CAD build for the part. Positions are in the model's coordinates, mm. Face numbers are marked on the shaded views. A direction names the side the tool comes from. Give positions to 0.01 mm unless a question says otherwise; leave off trailing zeros. Loops run counter-clockwise (first coordinate to the right, second up) from the corner with the lowest first, then second, coordinate; pieces in that order, holes last. Notation, with made-up numbers: (51.5, 64.25) - (91.5, 64.25) arc R17 ccw to (91.5, 92.25) - close; hole circle Ø1 at (55.25, 37.25). An arc over 180 degrees is marked (long way). Return JSON: item names as keys, results as strings.
from build123d import *

# Parameters (mm, degrees)
SKETCH1_R           = 6
SKETCH1_R_2         = 2.4
BOSS_EXTRUDE1_DEPTH = 20
SKETCH2_R           = 3.9
CUT_EXTRUDE1_DEPTH  = 7.5
CUT_EXTRUDE2_START  = -10
CUT_EXTRUDE2_DEPTH  = 10
FILLET1_R           = 1


with BuildPart() as part:
    # Sketch1 → Boss-Extrude1 (new body)
    with BuildSketch(Plane.XY):
        Circle(SKETCH1_R)
        Circle(SKETCH1_R_2, mode=Mode.SUBTRACT)
    extrude(amount=BOSS_EXTRUDE1_DEPTH)

    # Sketch2 → Cut-Extrude1 (cut)
    with BuildSketch(Plane.XY.offset(20)):
        Circle(SKETCH2_R)
    extrude(amount=-CUT_EXTRUDE1_DEPTH, mode=Mode.SUBTRACT)

    # Sketch4 → Cut-Extrude2 (cut)
    with BuildSketch(Plane.XY.offset(20).offset(CUT_EXTRUDE2_START)):
        with BuildLine():
            Line((-2.397915762, 5.5), (2.397915762, 5.5))
            ThreePointArc((2.397915762, 5.5), (0, 6), (-2.397915762, 5.5))
        make_face()
        with BuildLine():
            Line((2.397915762, -5.5), (-2.397915762, -5.5))
            ThreePointArc((-2.397915762, -5.5), (0, -6), (2.397915762, -5.5))
        make_face()
    extrude(amount=CUT_EXTRUDE2_DEPTH, mode=Mode.SUBTRACT)

    # Fillet1
    fillet1_edges = [part.edges().sort_by_distance(p)[0] for p in [
        (-2.397915762, 5.5, 15),
        (2.397915762, 5.5, 15),
        (2.397915762, -5.5, 15),
        (-2.397915762, -5.5, 15),
    ]]
    fillet(fillet1_edges, radius=FILLET1_R)


solid = part.part
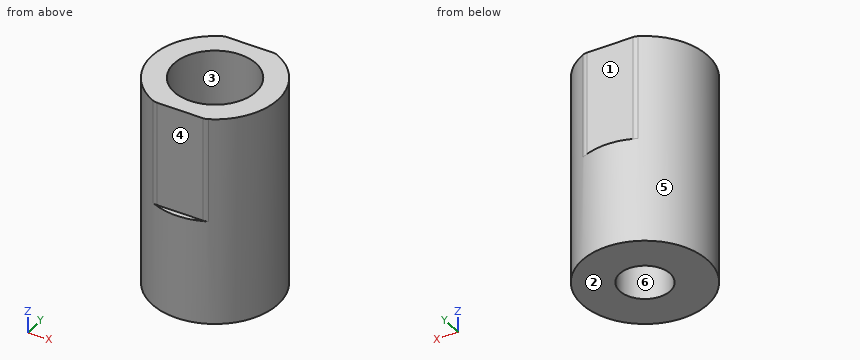
1. Which spindle directions (+Z, -Z, +X, -X, +Y, -Y) get a long thin tool onto all of the face, cutting with end or side? Do the marked faces 1, 2 and 3. Say none if no direction does.
Values follow:
{"face 1": "+Z, +X, -X, +Y", "face 2": "-Z, +X, -X, +Y, -Y", "face 3": "+Z"}
2. Cut at B-B, the plane x = 0. Write the cut outline in (y, z), plus the area to 4 significant figures.
Values follow:
{"outline": "(-6, 0) - (-2.4, 0) - (-2.4, 12.5) - (-3.9, 12.5) - (-3.9, 20) - (-5.5, 20) - (-5.5, 10) - (-6, 10) - close; (2.4, 0) - (6, 0) - (6, 10) - (5.5, 10) - (5.5, 20) - (3.9, 20) - (3.9, 12.5) - (2.4, 12.5) - close", "area": "111.5 mm²"}
3. Drill centre lines: probe 1 along Y at (x, z) = (0, 16.5); probe 2 along Y at (x, z) = (0, 8.5). Where is each one in solid material? Low to high.
Values follow:
{"probe 1": "y = -5.5 to -3.9, 3.9 to 5.5", "probe 2": "y = -6 to -2.4, 2.4 to 6"}
4. Cut at C-C, the plane y = 0. Write the cut outline in (x, z).
Values follow:
{"outline": "(-6, 0) - (-2.4, 0) - (-2.4, 12.5) - (-3.9, 12.5) - (-3.9, 20) - (-6, 20) - close; (2.4, 0) - (6, 0) - (6, 20) - (3.9, 20) - (3.9, 12.5) - (2.4, 12.5) - close"}
5. Pull direction Y, two halves, no side cores. Call the marked faces 4, 5 and 6: +Y half, -Y half, draft (parallel to the pull), parting line (faces both ways), or undercut.
Values follow:
{"face 4": "-Y half", "face 5": "parting line", "face 6": "undercut"}
6. Drop flat-ended pins along their axis: P1, Ø1, axis at x = 3, z = 2, coming from the +Y side; P2, Ø5, axis at x = 4, y = -3.5, coming from the -Z side; P3, Ø1, axis at x = 2, y = 0, coming from the +Z side; P4, Ø1.5, axis at y = -2, z = 16, coming from the -X side. Give the stop position or say it passes through.
Values follow:
{"P1": "stops at y = 5.45", "P2": "stops at z = 0", "P3": "stops at z = 12.5", "P4": "stops at x = -5.87"}
7. Cut at D-D, the plane y = -2.75. Write the cut outline in (x, z).
Values follow:
{"outline": "(-5.33, 0) - (5.33, 0) - (5.33, 20) - (2.77, 20) - (2.77, 12.5) - (-2.77, 12.5) - (-2.77, 20) - (-5.33, 20) - close"}
8. Cut at A-A, the plane z = 15.5. Write the cut outline in (x, y).
Values follow:
{"outline": "(-2.62, -5.4) arc R1 ccw to (-2.18, -5.5) - (2.18, -5.5) arc R1 ccw to (2.62, -5.4) arc R6 ccw to (2.62, 5.4) arc R1 ccw to (2.18, 5.5) - (-2.18, 5.5) arc R1 ccw to (-2.62, 5.4) arc R6 ccw to start; hole circle Ø7.8 at (0, 0)"}
